from build123d import *

# Parameters (mm, degrees)
SKETCH1_R           = 4.1
SKETCH1_R_2         = 4
BOSS_EXTRUDE1_DEPTH = 2
SKETCH3_R           = 7.5
BOSS_EXTRUDE3_DEPTH = 11
SKETCH4_R           = 2.5
CUT_EXTRUDE1_DEPTH  = 48.436800061


with BuildPart() as part:
    # Sketch1 → Boss-Extrude1 (new body)
    with BuildSketch(Plane(origin=(0, 0, 0), x_dir=(1, 0, 0), z_dir=(0, 1, 0))):
        with BuildLine():
            Line((-37.5, 7.5), (37.5, 7.5))
            ThreePointArc((37.5, 7.5), (45, 0), (37.5, -7.5))
            Line((37.5, -7.5), (-37.5, -7.5))
            ThreePointArc((-37.5, -7.5), (-45, 0), (-37.5, 7.5))
        make_face()
        with Locations(Location((-37.5, 0, 0), (0, 0, 270))):
            Circle(SKETCH1_R, mode=Mode.SUBTRACT)
        with Locations(Location((37.5, 0, 0), (0, 0, 270))):
            Circle(SKETCH1_R_2, mode=Mode.SUBTRACT)
    extrude(amount=BOSS_EXTRUDE1_DEPTH)

    # Sketch3 → Boss-Extrude3 (add)
    with BuildSketch(Plane(origin=(0, 2, 0), x_dir=(1, 0, 0), z_dir=(0, 1, 0))):
        with Locations(Location((0, 0, 0), (0, 0, 270))):
            Circle(SKETCH3_R)
    extrude(amount=BOSS_EXTRUDE3_DEPTH)

    # Sketch4 → Cut-Extrude1 (cut, through all)
    with BuildSketch(Plane(origin=(0, 13, 0), x_dir=(1, 0, 0), z_dir=(0, 1, 0))):
        with Locations(Location((0, 0, 0), (0, 0, 270))):
            Circle(SKETCH4_R)
    extrude(amount=-CUT_EXTRUDE1_DEPTH, mode=Mode.SUBTRACT)


solid = part.part
Geometry check sheet. Reference: the model listing, model coordinates, mm. Give positions to 0.01 mm unless a question says otherwise; leave off trailing zeros. Order: outer loops, then holes, each group sorted by start corner. A loop starts at its lowest first (then second) coordinate and runs counter-clockwise, first axis right, second up. Notation, with made-up numbers: M 60.25,87 L 106.25,87 A11 ccw 106.25,94 Z; hole C 53.25,34 d9. An arc over 180 degrees is marked long. Use a Markdown table: item, result.
Item 1: Section check B-B (y = 5.75). Record the cut outline in (x, z).
Answers follow:
| item | result |
|---|---|
| outline | C 0,0 d15; hole C 0,0 d5 |
Item 2: Section check A-A (z = 0). Record the cut outline in (x, y).
Answers follow:
| item | result |
|---|---|
| outline | M -45,0 L -41.6,0 L -41.6,2 L -45,2 Z; M -33.4,0 L -2.5,0 L -2.5,13 L -7.5,13 L -7.5,2 L -33.4,2 Z; M 2.5,0 L 33.5,0 L 33.5,2 L 7.5,2 L 7.5,13 L 2.5,13 Z; M 41.5,0 L 45,0 L 45,2 L 41.5,2 Z |
Item 3: Section check C-C (z = 6.5). Record the cut outline in (x, y), and give its area (3 significant figures).
Answers follow:
| item | result |
|---|---|
| outline | M -41.24,0 L 41.24,0 L 41.24,2 L 3.74,2 L 3.74,13 L -3.74,13 L -3.74,2 L -41.24,2 Z |
| area | 247 mm2 |
Item 4: Depth check by flat-ended pin: P1, Ø8, axis at x = 0, z = 0, coming from the +Y side; P2, Ø5, axis at y = 5, z = 4.5, coming from the +X side; P3, Ø1.5, axis at x = -5, y = 10, coming from the +Z side; P4, Ø5, axis at y = 10, z = -2, coming from the -X side. Enter the tip coordinate at first touch or a pass-through.
Answers follow:
| item | result |
|---|---|
| P1 | stops at y = 13 |
| P2 | stops at x = 7.23 |
| P3 | stops at z = 6.18 |
| P4 | stops at x = -7.5 |
Item 5: Draft check along X on faces 1 (the cylindrical face through (0.33, 7.423, -7.493)), 2 (the cylindrical face through (-45, 1, 0)), 3 (the cylindrical face through (41.466, 0.986, -0.521)). Enter one of: +X half, -X half, draft (parallel to the pull), parting line (faces both ways), or undercut.
Answers follow:
| item | result |
|---|---|
| face 1 | parting line |
| face 2 | -X half |
| face 3 | undercut |
Item 6: Section check D-D (x = 12.5). Record the cut outline in (y, z).
Answers follow:
| item | result |
|---|---|
| outline | M 0,-7.5 L 2,-7.5 L 2,7.5 L 0,7.5 Z |
Item 7: Material ranges on line 1 along X through (y, z) = (0.85, 0); line 2 along X through (y, z) = (3.25, 0); line 3 along Y through (x, z) = (-6.5, -4.5), recorded low to high.
Answers follow:
| item | result |
|---|---|
| line 1 | x = -45 to -41.6, -33.4 to -2.5, 2.5 to 33.5, 41.5 to 45 |
| line 2 | x = -7.5 to -2.5, 2.5 to 7.5 |
| line 3 | y = 0 to 2 |
